from build123d import *

# Parameters (mm, degrees)
BOSS_EXTRUDE1_DEPTH      = 7
BOSS_EXTRUDE1_DEPTH_BACK = 7
SKETCH2_R                = 3.0000000000000018
BOSS_EXTRUDE2_DEPTH      = 2
BOSS_EXTRUDE2_DEPTH_BACK = 2
SKETCH3_R                = 14.700000000000001
BOSS_EXTRUDE3_START      = 5
SKETCH4_R                = 14.700000000000001
SKETCH4_R_2              = 12.699999999999998
BOSS_EXTRUDE3_DEPTH      = 5
FILLET2_R                = 0.5
FILLET4_R                = 0.5
CHAMFER1_SIZE            = 0.5
CHAMFER2_SIZE            = 1


with BuildPart() as part:
    # Sketch2 → Boss-Extrude1 (new, two sides: drawn at the far end of the back side and taken through both)
    with BuildSketch(Plane.XY.offset(-BOSS_EXTRUDE1_DEPTH_BACK)):
        with BuildLine():
            Line((30.512377936980783, 70.89647327651264), (21.781878923827843, 61.0053372557492))
            ThreePointArc((21.781878923827843, 61.0053372557492), (13.313031061350836, 60.477496482202135), (12.78519028780376, 68.94634434467913))
            Line((12.78519028780376, 68.94634434467913), (21.51568930095671, 78.83748036544256))
            Line((21.51568930095671, 78.83748036544256), (30.512377936980783, 70.89647327651264))
        make_face()
        with Locations((17.283534605815802, 64.97584080021417)):
            Circle(SKETCH2_R, mode=Mode.SUBTRACT)
    extrude(amount=BOSS_EXTRUDE1_DEPTH + BOSS_EXTRUDE1_DEPTH_BACK)

    # Sketch3 → Boss-Extrude2 (add, two sides: drawn at the far end of the back side and taken through both)
    with BuildSketch(Plane(origin=(48.53568375746082, 54.98804239970119, 0), x_dir=(0.7497240530020064, -0.66175059074416, 0), z_dir=(0.66175059074416, 0.7497240530020064, 0)).offset(-BOSS_EXTRUDE2_DEPTH_BACK)):
        with Locations(Location((-30.039919418767553, 0, 0), (0, 0, 180))):
            Circle(SKETCH3_R)
    extrude(amount=BOSS_EXTRUDE2_DEPTH + BOSS_EXTRUDE2_DEPTH_BACK)

    # Sketch4 → Boss-Extrude3 (add)
    with BuildSketch(Plane(origin=(49.85918493894915, 56.48749050570521, 0), x_dir=(0.7497240530020064, -0.66175059074416, 0), z_dir=(0.66175059074416, 0.7497240530020064, 0)).offset(BOSS_EXTRUDE3_START)):
        with Locations(Location((-30.03991941876756, 0, 0), (0, 0, 180))):
            Circle(SKETCH4_R)
        with Locations(Location((-30.03991941876756, 0, 0), (0, 0, 180))):
            Circle(SKETCH4_R_2, mode=Mode.SUBTRACT)
    extrude(amount=-BOSS_EXTRUDE3_DEPTH)

    # Fillet2
    fillet2_edges = [part.edges().sort_by_distance(p)[0] for p in [
        (41.66723133330735, 70.38731150805249, 3.6e-15),
        (40.16778322730333, 71.7108126895408, 3.11e-15),
    ]]
    fillet(fillet2_edges, radius=FILLET2_R)

    # Fillet4
    fillet4_edges = [part.edges().sort_by_distance(p)[0] for p in [
        (13.313031061350841, 60.47749648220213, 7),
        (25.48537783966015, 65.2011812131289, 7),
        (16.488689203636067, 73.14218830205883, 7),
        (25.48537783966015, 65.2011812131289, -7),
        (16.488689203636067, 73.14218830205883, -7),
        (13.313031061350841, 60.47749648220213, -7),
    ]]
    fillet(fillet4_edges, radius=FILLET4_R)

    # Chamfer1
    chamfer1_edges = [part.edges().sort_by_distance(p)[0] for p in [
        (14.2835346058158, 64.97584080021417, -7),
        (14.2835346058158, 64.97584080021417, 7),
    ]]
    chamfer(chamfer1_edges, length=CHAMFER1_SIZE)

    # Chamfer2
    chamfer2_edges = [part.edges().sort_by_distance(p)[0] for p in [
        (35.711476016609915, 63.639795031034424, 3.6e-15),
        (24.690532437480417, 73.36752871497357, -7),
        (29.188876755492455, 69.39702517050861, -2.2e-16),
        (20.192188119468376, 77.33803225943853, -2.2e-16),
        (24.690532437480417, 73.36752871497357, 7),
        (29.079082209939642, 69.493936300796, -6.853553390593275),
        (20.301982665021182, 77.24112112915115, -6.853553390593271),
        (29.079082209939642, 69.493936300796, 6.853553390593275),
        (20.301982665021182, 77.24112112915115, 6.853553390593271),
    ]]
    chamfer(chamfer2_edges, length=CHAMFER2_SIZE)


solid = part.part
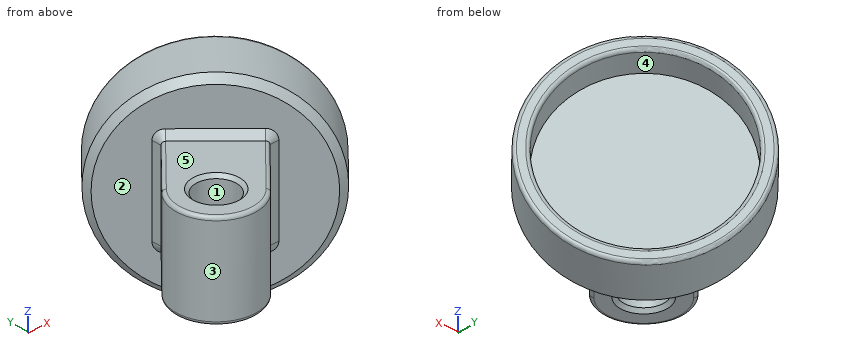
Can you work these out from the model? Positions are in its coordinate system, mm. Face numbers are marked on the shaded views. A direction names the side the tool comes from. Give positions to 0.01 mm unless a question says otherwise; leave off trailing zeros. Return JSON: item names as keys, results as strings.
Q1. I want a section at A-A, the plane y = 66.5. Count the separate pieces of the cut face and the enclosed holes in it, then the cut area to 3 significant figures.
Checks:
{"separate pieces": "3", "enclosed holes": "0", "area": "219 mm2"}
Q2. We'd pull the mould along X, two halves only. Please class the marked faces 3, 4 and 5: released by +X, released by -X, zero draft, split by the parting line, or undercut.
Checks:
{"face 3": "split by the parting line", "face 4": "undercut", "face 5": "zero draft"}
Q3. I need wall thicknesses on probe 1 along Z at (x, y) = (32, 77); probe 2 along Z at (x, y) = (27, 82.5); probe 3 along X at (y, z) = (72, -9.25). Which ranges of each line are inside material? Lowest first, please.
Checks:
{"probe 1": "z = -14.37 to -12.32, 12.32 to 14.37", "probe 2": "z = -14.05 to -11.95, 11.95 to 14.05", "probe 3": "x = 26.24 to 32.28, 35.09 to 38.72"}
Q4. On a 3-axis mill with a long thin cutter (end or side, diameter ignored), from which of +Z, -Z, +X, -X, +Y, -Y can I reach the whole of each face in a straight line? I mean the marked faces 1 and 2. Say none if no direction works.
Checks:
{"face 1": "+Z, -Z", "face 2": "none"}
Q5. For pin 1 Ø12 at (x, z) = (24.5, 9) entering from +Y; pin 2 Ø12 at (x, z) = (26, -8) entering from +Y; pin 3 Ø1 at (x, z) = (14.5, 1.5) entering from -Y, each with a flat end and sliding along its axis, tell me the tip position at first contact or that it passes through.
Checks:
{"pin 1": "stops at y = 89.12", "pin 2": "stops at y = 88.92", "pin 3": "stops at y = 59.43"}
